For this review, use the dimensioned drawing (mm, ordinates from the lowest corner) and the shaded views. A direction names the side the tool comes from. Give positions to 0.01 mm unless a question says otherwise; leave off trailing zeros. Loops run counter-clockwise (first coordinate to the right, second up) from the corner with the lowest first, then second, coordinate; pieces in that order, holes last. Notation, with made-up numbers: (41, 6) - (90, 6) arc R13 ccw to (90, 23) - close; hole circle Ø9 at (5, 89). An arc over 180 degrees is marked (long way). Put each result on its own line as item: value.
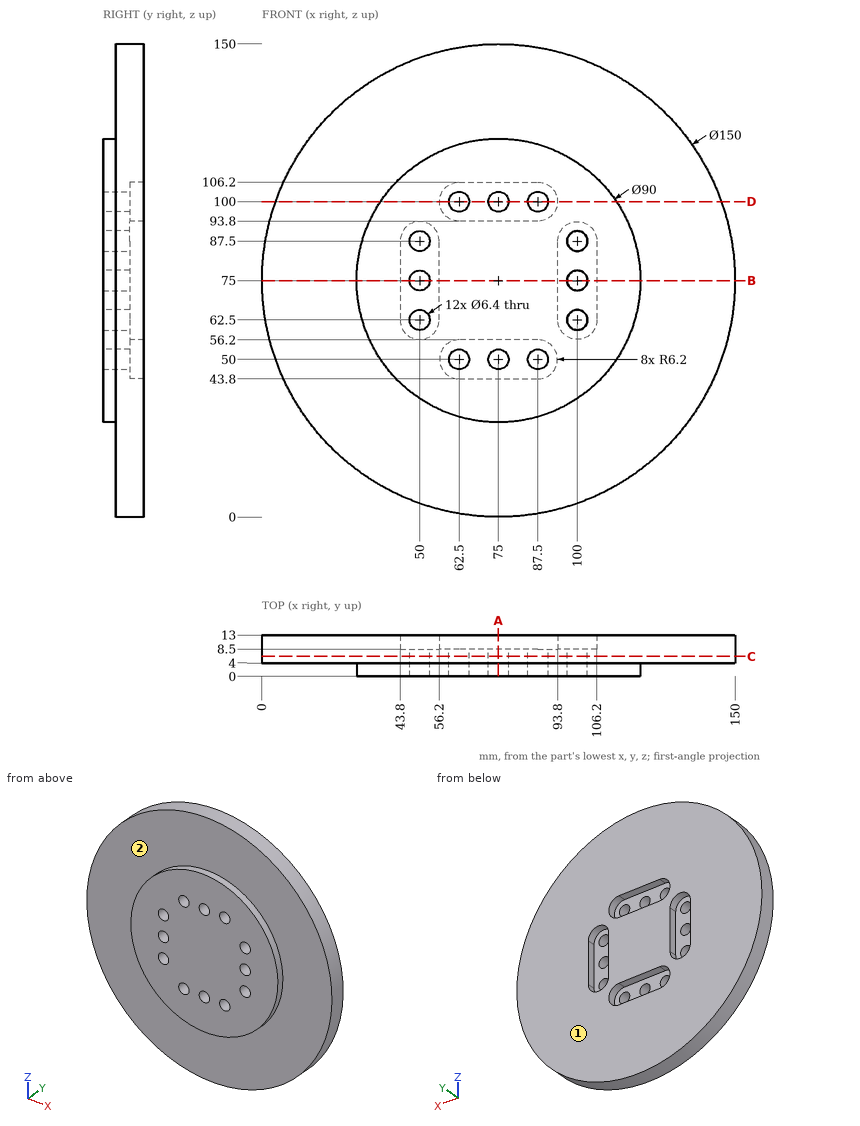
1) Take a section at A-A on x = 75. State the section outline as (y, z) points, and give its area (3 significant figures).
Geometry check:
outline: (0, 30) - (4, 30) - (4, 0) - (13, 0) - (13, 43.8) - (8.5, 43.8) - (8.5, 46.8) - (0, 46.8) - close; (0, 53.2) - (8.5, 53.2) - (8.5, 56.2) - (13, 56.2) - (13, 93.8) - (8.5, 93.8) - (8.5, 96.8) - (0, 96.8) - close; (0, 103.2) - (8.5, 103.2) - (8.5, 106.2) - (13, 106.2) - (13, 150) - (4, 150) - (4, 120) - (0, 120) - close
area: 1,490 mm²
2) Wall thickness on line 1 (X direction, y = 2, z = 62.5); line 2 (X direction, y = 8.25, z = 51); line 3 (X direction, y = 5.75, z = 52): over which ranges is each line inside the solid? List them lowest first.
Geometry check:
line 1: x = 31.77 to 46.8, 53.2 to 96.8, 103.2 to 118.23
line 2: x = 3.94 to 59.46, 65.54 to 71.96, 78.04 to 84.46, 90.54 to 146.06
line 3: x = 3.61 to 60, 65 to 72.5, 77.5 to 85, 90 to 146.39
3) For the marked faces 1 and 2, list the 3-axis set-ups (+Z, -Z, +X, -X, +Y, -Y) from which the entire face can be reached by the end or side of a thin tool; tool diameter is ignored.
Geometry check:
face 1: +Z, -Z, +X, -X, +Y
face 2: -Y
4) Take a section at C-C on y = 6.25. State how many separate pieces and enclosed holes the cut face has, and give its area (3 significant figures).
Geometry check:
separate pieces: 1
enclosed holes: 12
area: 17,300 mm²
5) Insertion check: pin 1 Ø1.3 at (y, z) = (11, 80.5) entering from -X; pin 2 Ø3.5 at (y, z) = (10, 80) entering from -X; pin 3 Ø2 at (y, z) = (10, 78.5) entering from +X. Each pin has a flat end and moves straight along its axis. Give the tip position at first contact, or say it passes through.
Geometry check:
pin 1: stops at x = 0.16
pin 2: stops at x = 0.07
pin 3: stops at x = 149.96
6) Take a section at B-B on z = 75. State the section outline as (x, y) points.
Geometry check:
outline: (0, 4) - (30, 4) - (30, 0) - (46.8, 0) - (46.8, 8.5) - (43.8, 8.5) - (43.8, 13) - (0, 13) - close; (53.2, 0) - (96.8, 0) - (96.8, 8.5) - (93.8, 8.5) - (93.8, 13) - (56.2, 13) - (56.2, 8.5) - (53.2, 8.5) - close; (103.2, 0) - (120, 0) - (120, 4) - (150, 4) - (150, 13) - (106.2, 13) - (106.2, 8.5) - (103.2, 8.5) - close
7) Take a section at D-D on z = 100. State the section outline as (x, y) points.
Geometry check:
outline: (4.29, 4) - (37.58, 4) - (37.58, 0) - (59.3, 0) - (59.3, 8.5) - (56.3, 8.5) - (56.3, 13) - (4.29, 13) - close; (65.7, 0) - (71.8, 0) - (71.8, 8.5) - (65.7, 8.5) - close; (78.2, 0) - (84.3, 0) - (84.3, 8.5) - (78.2, 8.5) - close; (90.7, 0) - (112.42, 0) - (112.42, 4) - (145.71, 4) - (145.71, 13) - (93.7, 13) - (93.7, 8.5) - (90.7, 8.5) - close
